Autodesk Fusion 360 part; units mm, degrees
sketch "Skizze1" plane through (0, 0, 0) normal (0, 1, 0) x (1, 0, 0)
  line L0 (108, 39) -> (-108, 39)
  line L1 (-108, 39) -> (-108, -39)
  line L2 (-108, -39) -> (108, -39)
  line L3 (108, -39) -> (108, 39)
  line L4 (108, 39) -> (-108, -39) construction
  line L5 (-108, 39) -> (108, -39) construction
  line L6 (109, 40) -> (-109, 40)
  line L7 (-109, 40) -> (-109, -40)
  line L8 (-109, -40) -> (109, -40)
  line L9 (109, -40) -> (109, 40)
  line L10 (109, 40) -> (-109, -40) construction
  line L11 (-109, 40) -> (109, -40) construction
  dimension "d4" = 216
  dimension "d5" = 78
  dimension "d6" = 218
  dimension "d7" = 80
extrude "Extrusion1" add sketch "Skizze1" along normal blind 1 contours L0 L1 L2 L3 | L6 L7 L8 L9
extrude "Extrusion2" add sketch "Skizze1" along normal blind 51
Input: part model. Units: mm. Frame: model coordinates. A direction names the side the tool comes from. Give positions to 0.01 mm unless a question says otherwise; leave off trailing zeros. Order: outer loops, then holes, each group sorted by start corner. A loop starts at its lowest first (then second) coordinate and runs counter-clockwise, first axis right, second up.
1. Set-up query: faces 5 (the face through (-2, 25, 40)), 6 (the face through (2, 26, -39)). Return all of +Z, -Z, +X, -X, +Y, -Y with unobstructed straight access to the full face (end or side cutting, diameter ignored); none if empty.
Computed:
face 5: +Z, +X, -X, +Y, -Y
face 6: +Y
2. Draft query along X for faces 1 (the face through (-2, 26, 39)), 2 (the face through (-109, 25, -1)), 3 (the face through (109, 25, 1)), 4 (the face through (108, 26, 1)). Return one class per face: released by +X, released by -X, zero draft, split by the parting line, or undercut.
Computed:
face 1: undercut
face 2: released by -X
face 3: released by +X
face 4: undercut
3. Cut plane C-C (x = 56). Return loops of the section in (y, z), and give its area (3 significant figures).
Computed:
outline: (0, -40) - (51, -40) - (51, -39) - (1, -39) - (1, 39) - (51, 39) - (51, 40) - (0, 40) - close
area: 180 mm2
4. Cut plane B-B (z = 19.5). Return loops of the section in (x, y), and give its area (3 significant figures).
Computed:
outline: (-109, 0) - (109, 0) - (109, 51) - (108, 51) - (108, 1) - (-108, 1) - (-108, 51) - (-109, 51) - close
area: 318 mm2
5. Line query: probe 1 along Z at (x, y) = (-34.5, 29); probe 2 along X at (y, z) = (31, -11.5); probe 3 along Y at (x, z) = (-97.5, -25). Output: solid intervals per line, ascending.
Computed:
probe 1: z = -40 to -39, 39 to 40
probe 2: x = -109 to -108, 108 to 109
probe 3: y = 0 to 1
6. Cut plane A-A (y = 25). Return loops of the section in (x, z).
Computed:
outline: (-109, -40) - (109, -40) - (109, 40) - (-109, 40) - close; hole (-108, -39) - (108, -39) - (108, 39) - (-108, 39) - close
7. Pin query (flat end, axial travel): pin 1 Ø23.5 at (x, z) = (16.5, 10) entering from +Y. Return the tip coordinate at first contact, or that it passes through.
Computed:
pin 1: stops at y = 1
